Geometry check sheet. Reference: the model listing, model coordinates, mm. Face numbers are marked on the shaded views. A direction names the side the tool comes from. Coordinates: 2 decimals unless noted, no trailing zeros. Write each loop counter-clockwise with the first axis right and the second up, starting at its lowest first coordinate (ties: lowest second). Pieces come first, ordered by that corner, then holes. Notation, with made-up numbers: M 67,38 L 81,38 A14 cw 81,54 Z; hole C 3,-39.5 d2. An arc over 180 degrees is marked long. Put each result on its own line as item: value. Start each with the question number.
1) Mould release check, pull along Y, two halves, no side actions. Record for the marked faces 1, 2 and 3: released by +Y, released by -Y, zero draft, split by the parting line, or undercut.
2) Gauge pin test, flat ends, axial feed: pin 1 (6 mm diameter, centred on y = -15.5, z = 6.5, fed in from -X); pin 2 (7 mm diameter, centred on x = 33.35, z = 0, fed in from -Y); pin 3 (5.5 mm diameter, centred on x = 4, z = 36.5, fed in from +Y). Record the tip position at first contact, or that the pin passes through.
3) Scan lines: line 1 along X through (y, z) = (3.35, 0); line 2 along Z through (x, y) = (-20.5, -14); line 3 along X through (y, z) = (-80, -2). Record each from-to range of solid material in increasing order.
4) Cross-section at A-A on z = 0. Record the cut outline in (x, y).
5) Cross-section at C-C on z = 39. Record the cut outline in (x, y).
6) Set-up check for the marked faces 4, 5, 6, 7 and 8: record each of +Z, -Z, +X, -X, +Y, -Y from which the full face is reachable in a straight line by a thin tool's end or side.
7) Cross-section at B-B on y = -25.5. Record the cut outline in (x, z), plus the area to 3 significant figures.
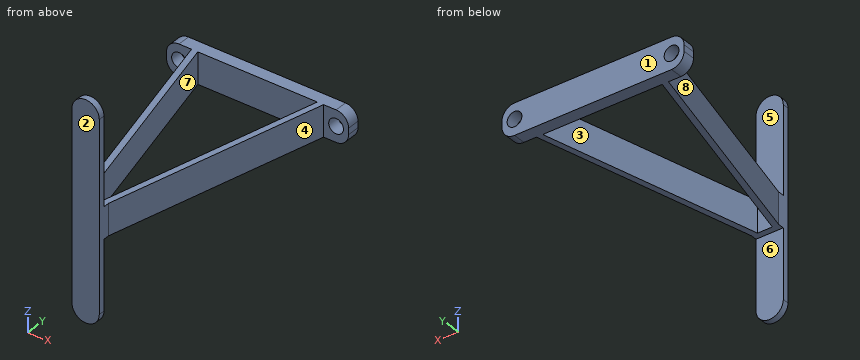
from build123d import *

# Parameters (mm, degrees)
SKETCH1_R           = 3
BOSS_EXTRUDE1_DEPTH = 5.08
BOSS_EXTRUDE2_DEPTH = 12.7
BOSS_EXTRUDE3_DEPTH = 2.54


with BuildPart() as part:
    # Sketch1 → Boss-Extrude1 (new body)
    with BuildSketch(Plane(origin=(0, 0, 0), x_dir=(1, 0, 0), z_dir=(0, 1, 0))):
        with BuildLine():
            Line((-24.747623202, 6.35), (-30.399794039, 6.35))
            ThreePointArc((-30.399794039, 6.35), (-33.991896487, 4.862102448), (-35.479794039, 1.27))
            Line((-35.479794039, 1.27), (-35.479794039, -1.27))
            ThreePointArc((-35.479794039, -1.27), (-33.991896487, -4.862102448), (-30.399794039, -6.35))
            Line((-30.399794039, -6.35), (-24.747623202, -6.35))
            Line((-24.747623202, -6.35), (27.702035125, -6.35))
            Line((27.702035125, -6.35), (33.354205961, -6.35))
            ThreePointArc((33.354205961, -6.35), (36.94630841, -4.862102448), (38.434205961, -1.27))
            Line((38.434205961, -1.27), (38.434205961, 1.27))
            ThreePointArc((38.434205961, 1.27), (36.94630841, 4.862102448), (33.354205961, 6.35))
            Line((33.354205961, 6.35), (27.702035125, 6.35))
            Line((27.702035125, 6.35), (-24.747623202, 6.35))
        make_face()
        with Locations(Location((-30.399794039, 0, 0), (0, 0, 270))):
            Circle(SKETCH1_R, mode=Mode.SUBTRACT)
        with Locations(Location((33.354205961, 0, 0), (0, 0, 270))):
            Circle(SKETCH1_R, mode=Mode.SUBTRACT)
    extrude(amount=BOSS_EXTRUDE1_DEPTH)

    # Sketch3 → Boss-Extrude2 (add)
    with BuildSketch(Plane.XY.offset(6.35)):
        Polygon((-25.319794039, 0), (-4.062794039, -87.74317324), (-4.062794039, -90.28317324), (7.017205961, -90.28317324), (7.017205961, -87.74317324), (28.274205961, 0), (25.734205961, 0), (4.477205961, -87.74317324), (-1.522794039, -87.74317324), (-22.779794039, 0), align=None)
    extrude(amount=-BOSS_EXTRUDE2_DEPTH)

    # Sketch4 → Boss-Extrude3 (add)
    with BuildSketch(Plane.XZ.offset(90.28317324)):
        with BuildLine():
            Line((-4.062794039, 41.80872522), (-4.062794039, -34.39127478))
            ThreePointArc((-4.062794039, -34.39127478), (1.477205961, -39.93127478), (7.017205961, -34.39127478))
            Line((7.017205961, -34.39127478), (7.017205961, 41.80872522))
            ThreePointArc((7.017205961, 41.80872522), (1.477205961, 47.34872522), (-4.062794039, 41.80872522))
        make_face()
    extrude(amount=BOSS_EXTRUDE3_DEPTH)


solid = part.part
Answer key:
1. face 1: released by +Y
1. face 2: released by -Y
1. face 3: undercut
2. pin 1: stops at x = -22.29
2. pin 2: stops at y = 0
2. pin 3: stops at y = -90.28
3. line 1: x = -35.48 to -33.4, -27.4 to 30.35, 36.35 to 38.43
3. line 2: z = -6.35 to 6.35
3. line 3: x = -5.94 to -3.4, 6.35 to 8.89
4. outline: M -35.48,0 L -33.4,0 L -33.4,5.08 L -35.48,5.08 Z; M -27.4,0 L -25.32,0 L -4.06,-87.74 L -4.06,-92.82 L 7.02,-92.82 L 7.02,-87.74 L 28.27,0 L 30.35,0 L 30.35,5.08 L -27.4,5.08 Z; M 36.35,0 L 38.43,0 L 38.43,5.08 L 36.35,5.08 Z; hole M -22.78,0 L -1.52,-87.74 L 4.48,-87.74 L 25.73,0 Z
5. outline: M -4.06,-92.82 L 7.02,-92.82 L 7.02,-90.28 L -4.06,-90.28 Z
6. face 4: +Z, -Z, +X, -Y
6. face 5: +Z, +X, -X, +Y
6. face 6: -Z, +X, -X, +Y
6. face 7: +Z, -Z
6. face 8: +Z, -Z, -X, -Y
7. outline: M -19.14,-6.35 L -16.6,-6.35 L -16.6,6.35 L -19.14,6.35 Z; M 19.56,-6.35 L 22.1,-6.35 L 22.1,6.35 L 19.56,6.35 Z
7. area: 64.5 mm²
